Input: part model. Units: mm. Frame: model coordinates. A direction names the side the tool comes from. Coordinates: 2 decimals unless noted, no trailing zeros. Write each loop counter-clockwise with the first axis right and the second up, starting at its lowest first coordinate (ties: lowest second). Pieces come first, ordered by that corner, then holes. Notation, with made-up numbers: (80, 51.25) - (117, 51.25) arc R9 ccw to (117, 65.25) - close; hole circle Ø11 at (-24, -36). An arc over 180 degrees is marked (long way). Use CSV: the item, a comma, the result in double quotes.
```python
from build123d import *

# Parameters (mm, degrees)
F0_R          = 1.080022686
F1_DEPTH      = 3.0734
F1_DEPTH_BACK = 3.0734
F2_R          = 1.0822492619
F3_DEPTH      = 3.0734
F3_DEPTH_BACK = 3.0734
F4_R          = 1.4624555287
F5_DEPTH      = 0.254
F6_R          = 1.4618158242
F7_DEPTH      = 0.254
F8_R          = 1.4581045409
F9_DEPTH      = 0.254
F10_R         = 1.4573675157
F11_DEPTH     = 0.254


with BuildPart() as f1:
    # F0 (on Front) → F1 (new body, two sides)
    with BuildSketch(Plane.XZ) as f1_sk:
        Circle(F0_R)
    extrude(amount=F1_DEPTH)
    extrude(f1_sk.sketch, amount=-F1_DEPTH_BACK)

    # F2 (on Right) → F3 (join, two sides)
    with BuildSketch(Plane.YZ) as f3_sk:
        Circle(F2_R)
    extrude(amount=F3_DEPTH)
    extrude(f3_sk.sketch, amount=-F3_DEPTH_BACK)

    # F4 (on face) → F5 (join)
    with BuildSketch(Plane.XZ.offset(3.0734)):
        Circle(F4_R)
    extrude(amount=F5_DEPTH)

    # F6 (on face) → F7 (join)
    with BuildSketch(Plane.YZ.offset(3.0734)):
        Circle(F6_R)
    extrude(amount=F7_DEPTH)

    # F8 (on face) → F9 (join)
    with BuildSketch(Plane(origin=(0, 3.0734, 0), x_dir=(-1, 0, 0), z_dir=(0, 1, 0))):
        Circle(F8_R)
    extrude(amount=F9_DEPTH)

    # F10 (on face) → F11 (join)
    with BuildSketch(Plane(origin=(-3.0734, 0, 0), x_dir=(0, -1, 0), z_dir=(-1, 0, 0))):
        Circle(F10_R)
    extrude(amount=F11_DEPTH)


solid = f1.part
```
(1) Cut plane D-D on z = 0.45. Return loops of the section in (x, y).
Check values:
outline,"(-3.33, -1.39) - (-3.07, -1.39) - (-3.07, -0.98) - (-0.98, -0.98) - (-0.98, -3.07) - (-1.39, -3.07) - (-1.39, -3.33) - (1.39, -3.33) - (1.39, -3.07) - (0.98, -3.07) - (0.98, -0.98) - (3.07, -0.98) - (3.07, -1.39) - (3.33, -1.39) - (3.33, 1.39) - (3.07, 1.39) - (3.07, 0.98) - (0.98, 0.98) - (0.98, 3.07) - (1.39, 3.07) - (1.39, 3.33) - (-1.39, 3.33) - (-1.39, 3.07) - (-0.98, 3.07) - (-0.98, 0.98) - (-3.07, 0.98) - (-3.07, 1.39) - (-3.33, 1.39) - close"
(2) Cut plane B-B on z = 0. Return loops of the section in (x, y), and give its area (3 significant figures).
Check values:
outline,"(-3.33, -1.46) - (-3.07, -1.46) - (-3.07, -1.08) - (-1.08, -1.08) - (-1.08, -3.07) - (-1.46, -3.07) - (-1.46, -3.33) - (1.46, -3.33) - (1.46, -3.07) - (1.08, -3.07) - (1.08, -1.08) - (3.07, -1.08) - (3.07, -1.46) - (3.33, -1.46) - (3.33, 1.46) - (3.07, 1.46) - (3.07, 1.08) - (1.08, 1.08) - (1.08, 3.07) - (1.46, 3.07) - (1.46, 3.33) - (-1.46, 3.33) - (-1.46, 3.07) - (-1.08, 3.07) - (-1.08, 1.08) - (-3.07, 1.08) - (-3.07, 1.46) - (-3.33, 1.46) - close"
area,"24.9 mm^2"
(3) Ray query, probe 1 along Y at (x, z) = (0.75, 1.2); probe 2 along Z at (x, y) = (0, 0.75); probe 3 along Y at (x, z) = (2.5, 0.35). Return the intervals inside material, ascending. Write a range as from..to.
Check values:
probe 1,"-3.33..-3.07, 3.07..3.33"
probe 2,"-1.08..1.08"
probe 3,"-1.02..1.02"
(4) Cut plane C-C on y = -1. Return loops of the section in (x, z), and give its area (3 significant figures).
Check values:
outline,"(-3.33, -1.06) - (-3.07, -1.06) - (-3.07, -0.41) - (-1, -0.41) arc R1.08 ccw to (1, -0.41) - (3.07, -0.41) - (3.07, -1.07) - (3.33, -1.07) - (3.33, 1.07) - (3.07, 1.07) - (3.07, 0.41) - (1, 0.41) arc R1.08 ccw to (-1, 0.41) - (-3.07, 0.41) - (-3.07, 1.06) - (-3.33, 1.06) - close"
area,"8.09 mm^2"
(5) Pin query (flat end, axial travel): pin 1 Ø2 at (x, y) = (2, -2.5) entering from +Z. Return the tip coordinate at first contact, or that it passes through.
Check values:
pin 1,"z = 0.86"
(6) Cut plane A-A on x = 0. Return loops of the section in (y, z).
Check values:
outline,"(-3.33, -1.46) - (-3.07, -1.46) - (-3.07, -1.08) - (-0.07, -1.08) arc R1.08 ccw to (0.07, -1.08) - (3.07, -1.08) - (3.07, -1.46) - (3.33, -1.46) - (3.33, 1.46) - (3.07, 1.46) - (3.07, 1.08) - (0.07, 1.08) arc R1.08 ccw to (-0.07, 1.08) - (-3.07, 1.08) - (-3.07, 1.46) - (-3.33, 1.46) - close"
(7) Reachability of faces 5 (the flat face through (0, 3.327, 0)), 6 (the cylindrical face through (-0.73, 0.5, -0.96)) from +Z, -Z, +X, -X, +Y, -Y: full face, straight path, thin tool, end or side. Return the list, or none.
Check values:
face 5,"+Z, -Z, +X, -X, +Y"
face 6,"none"
(8) Draft query along X for faces 1 (the flat face through (3.327, 0, 0)), 2 (the flat face through (0, -3.327, 0)), 3 (the flat face through (-3.327, 0, 0)), 4 (the cylindrical face through (-1.08, -1.93, 0.05)). Return one class per face: pulls with the +X half, pulls with the -X half, needs draft (parallel to the pull), parting line crosses it, or undercut.
Check values:
face 1,"pulls with the +X half"
face 2,"needs draft"
face 3,"pulls with the -X half"
face 4,"undercut"
